The model under review builds one solid part; all positions refer to its coordinate system, in mm. Face numbers are marked on the shaded views. A direction names the side the tool comes from. Coordinates: 2 decimals unless noted, no trailing zeros. Order: outer loops, then holes, each group sorted by start corner. A loop starts at its lowest first (then second) coordinate and runs counter-clockwise, first axis right, second up. Notation, with made-up numbers: (-32, 30.5) -> (11, 30.5) arc R20 cw to (11, 48.5) -> close; hole circle Ø3 at (11.5, -10). An arc over 180 degrees is marked (long way). Answer as CSV lines item,"result". Start each with the question number.
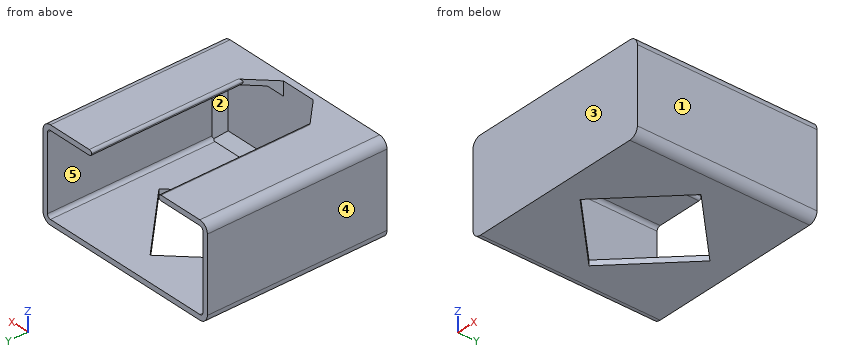
from build123d import *

# Parameters (mm, degrees)
RESSALTO_EXTRUS_O1_DEPTH = 1.5
RESSALTO_EXTRUS_O2_DEPTH = 40
ESBO_O4_W                = 18
ESBO_O4_H                = 3
CORTE_EXTRUS_O1_DEPTH    = 40
CORTE_EXTRUS_O2_DEPTH    = 8
CHANFRO1_SIZE            = 5
CHANFRO2_SIZE            = 2
FILETE2_START            = 6.5
FILETE2_DEPTH            = 35.5
FILETE2_START_2          = -3
FILETE2_2_DEPTH          = 1.232233047
FILETE3_START            = 6.5
FILETE3_DEPTH            = 35.5
FILETE3_START_2          = 1.767766953
FILETE3_2_DEPTH          = 1.232233047


with BuildPart() as part:
    # Esboço1 → Ressalto-extrusão1 (new body)
    with BuildSketch(Plane(origin=(0, 0, 0), x_dir=(1, 0, 0), z_dir=(0, 1, 0))):
        with BuildLine():
            Line((-20, -10.5), (20, -10.5))
            ThreePointArc((20, -10.5), (21.414213562, -9.914213562), (22, -8.5))
            Line((22, -8.5), (22, 8.5))
            ThreePointArc((22, 8.5), (21.414213562, 9.914213562), (20, 10.5))
            Line((20, 10.5), (-20, 10.5))
            ThreePointArc((-20, 10.5), (-21.414213562, 9.914213562), (-22, 8.5))
            Line((-22, 8.5), (-22, -8.5))
            ThreePointArc((-22, -8.5), (-21.414213562, -9.914213562), (-20, -10.5))
        make_face()
    extrude(amount=RESSALTO_EXTRUS_O1_DEPTH)

    # Esboço3 → Ressalto-extrusão2 (add)
    with BuildSketch(Plane(origin=(0, 1.5, 0), x_dir=(1, 0, 0), z_dir=(0, 1, 0))):
        with BuildLine():
            Line((-20, -10.5), (20, -10.5))
            ThreePointArc((20, -10.5), (21.414213562, -9.914213562), (22, -8.5))
            Line((22, -8.5), (22, 8.5))
            ThreePointArc((22, 8.5), (21.414213562, 9.914213562), (20, 10.5))
            Line((20, 10.5), (-20, 10.5))
            ThreePointArc((-20, 10.5), (-21.414213562, 9.914213562), (-22, 8.5))
            Line((-22, 8.5), (-22, -8.5))
            ThreePointArc((-22, -8.5), (-21.414213562, -9.914213562), (-20, -10.5))
        make_face()
        with BuildLine():
            Line((-20, 9.3), (20, 9.3))
            ThreePointArc((20, 9.3), (20.565685425, 9.065685425), (20.8, 8.5))
            Line((20.8, 8.5), (20.8, -8.5))
            ThreePointArc((20.8, -8.5), (20.565685425, -9.065685425), (20, -9.3))
            Line((20, -9.3), (-20, -9.3))
            ThreePointArc((-20, -9.3), (-20.565685425, -9.065685425), (-20.8, -8.5))
            Line((-20.8, -8.5), (-20.8, 8.5))
            ThreePointArc((-20.8, 8.5), (-20.565685425, 9.065685425), (-20, 9.3))
        make_face(mode=Mode.SUBTRACT)
    extrude(amount=RESSALTO_EXTRUS_O2_DEPTH)

    # Esboço4 → Corte-extrusão1 (cut)
    with BuildSketch(Plane(origin=(0, 41.5, 0), x_dir=(1, 0, 0), z_dir=(0, 1, 0))):
        with Locations((0, -9.3)):
            Rectangle(ESBO_O4_W, ESBO_O4_H)
    extrude(amount=-CORTE_EXTRUS_O1_DEPTH, mode=Mode.SUBTRACT)

    # Esboço5 → Corte-extrusão2 (cut)
    with BuildSketch(Plane(origin=(0, 0, -10.5), x_dir=(-1, 0, 0), z_dir=(0, 0, -1))):
        Polygon((0, 5.75), (15, 20.75), (0, 35.75), (-15, 20.75), align=None)
    extrude(amount=-CORTE_EXTRUS_O2_DEPTH, mode=Mode.SUBTRACT)

    # Chanfro1
    chanfro1_edges = [part.edges().sort_by_distance(p)[0] for p in [
        (9, 1.5, 9.9),
        (-9, 1.5, 9.9),
    ]]
    chamfer(chanfro1_edges, length=CHANFRO1_SIZE)

    # Chanfro2
    # the kernel refuses this chamfer: 2 mm, written as the material it adds along each edge
    with BuildSketch(Plane(origin=(-1.143365976, 1.5, 9.3), x_dir=(0, 1, 0), z_dir=(1, 0, 0))) as chanfro2_piece_1_section:
        Polygon((CHANFRO2_SIZE, 0), (0, -CHANFRO2_SIZE), (0, 0), align=None)
    chanfro2_piece_1 = extrude(amount=26.286731952, mode=Mode.PRIVATE)
    chanfro2_piece_1 = split(chanfro2_piece_1, bisect_by=Plane(origin=(20.8, 1.5, 9.3), z_dir=(-1, 0, 0)), keep=Keep.TOP, mode=Mode.PRIVATE)
    chanfro2_piece_1 = split(chanfro2_piece_1, bisect_by=Plane(origin=(1.428317012, -1.071682988, 9.3), z_dir=(0.7071067811865476, -0.7071067811865476, 0)), keep=Keep.TOP, mode=Mode.PRIVATE)
    add(chanfro2_piece_1)
    with BuildSketch(Plane(origin=(20.8, 1.5, -13.643365976), x_dir=(0, 1, 0), z_dir=(0, 0, 1))) as chanfro2_piece_2_section:
        Polygon((CHANFRO2_SIZE, 0), (0, CHANFRO2_SIZE), (0, 0), align=None)
    chanfro2_piece_2 = extrude(amount=27.286731952, mode=Mode.PRIVATE)
    chanfro2_piece_2 = split(chanfro2_piece_2, bisect_by=Plane(origin=(20.8, 1.5, -9.3), z_dir=(0, 0, 1)), keep=Keep.TOP, mode=Mode.PRIVATE)
    chanfro2_piece_2 = split(chanfro2_piece_2, bisect_by=Plane(origin=(20.8, 1.5, 9.3), z_dir=(0, 0, -1)), keep=Keep.TOP, mode=Mode.PRIVATE)
    add(chanfro2_piece_2)
    with BuildSketch(Plane(origin=(-25.143365976, 1.5, 9.3), x_dir=(0, 1, 0), z_dir=(1, 0, 0))) as chanfro2_piece_3_section:
        Polygon((CHANFRO2_SIZE, 0), (0, -CHANFRO2_SIZE), (0, 0), align=None)
    chanfro2_piece_3 = extrude(amount=26.286731952, mode=Mode.PRIVATE)
    chanfro2_piece_3 = split(chanfro2_piece_3, bisect_by=Plane(origin=(-20.8, 1.5, 9.3), z_dir=(1, 0, 0)), keep=Keep.TOP, mode=Mode.PRIVATE)
    chanfro2_piece_3 = split(chanfro2_piece_3, bisect_by=Plane(origin=(-14.571682988, 12.071682988, 9.3), z_dir=(-0.7071067811865476, -0.7071067811865476, 0)), keep=Keep.TOP, mode=Mode.PRIVATE)
    add(chanfro2_piece_3)
    with BuildSketch(Plane(origin=(-20.8, 1.5, 13.643365976), x_dir=(0, 1, 0), z_dir=(0, 0, -1))) as chanfro2_piece_4_section:
        Polygon((CHANFRO2_SIZE, 0), (0, CHANFRO2_SIZE), (0, 0), align=None)
    chanfro2_piece_4 = extrude(amount=27.286731952, mode=Mode.PRIVATE)
    chanfro2_piece_4 = split(chanfro2_piece_4, bisect_by=Plane(origin=(-20.8, 1.5, -9.3), z_dir=(0, 0, 1)), keep=Keep.TOP, mode=Mode.PRIVATE)
    chanfro2_piece_4 = split(chanfro2_piece_4, bisect_by=Plane(origin=(-20.8, 1.5, 9.3), z_dir=(0, 0, -1)), keep=Keep.TOP, mode=Mode.PRIVATE)
    add(chanfro2_piece_4)
    with BuildSketch(Plane(origin=(-25.143365976, 1.5, -9.3), x_dir=(0, 1, 0), z_dir=(1, 0, 0))) as chanfro2_piece_5_section:
        Polygon((CHANFRO2_SIZE, 0), (0, CHANFRO2_SIZE), (0, 0), align=None)
    chanfro2_piece_5 = extrude(amount=50.286731952, mode=Mode.PRIVATE)
    chanfro2_piece_5 = split(chanfro2_piece_5, bisect_by=Plane(origin=(20.8, 1.5, -9.3), z_dir=(-1, 0, 0)), keep=Keep.TOP, mode=Mode.PRIVATE)
    chanfro2_piece_5 = split(chanfro2_piece_5, bisect_by=Plane(origin=(-20.8, 1.5, -9.3), z_dir=(1, 0, 0)), keep=Keep.TOP, mode=Mode.PRIVATE)
    add(chanfro2_piece_5)
    with BuildSketch(Plane(origin=(-20, 1.5, -8.5), x_dir=(-1, 0, 0), z_dir=(0, 0, 1))) as chanfro2_piece_6_section:
        Polygon((0.8, -CHANFRO2_SIZE), (0, -1.2), (0, 0), (0.8, 0), align=None)
    chanfro2_piece_6 = revolve(axis=Axis((-20, 1.5, -8.5), (0, -1, 0)), revolution_arc=90, mode=Mode.PRIVATE)
    chanfro2_piece_6 = split(chanfro2_piece_6, bisect_by=Plane(origin=(-19.4, 2.1, -8.5), z_dir=(-0.7071067811865476, -0.7071067811865476, 0)), keep=Keep.TOP, mode=Mode.PRIVATE)
    add(chanfro2_piece_6)
    with BuildSketch(Plane(origin=(-20, 1.5, -8.5), x_dir=(-1, 0, 0), z_dir=(0, 0, 1))) as chanfro2_piece_7_section:
        Polygon((0.8, -CHANFRO2_SIZE), (0, -1.2), (0, 0), (0.8, 0), align=None)
    chanfro2_piece_7 = revolve(axis=Axis((-20, 1.5, -8.5), (0, -1, 0)), revolution_arc=90, mode=Mode.PRIVATE)
    chanfro2_piece_7 = split(chanfro2_piece_7, bisect_by=Plane(origin=(-20, 2.1, -7.9), z_dir=(0, -0.7071067811865476, -0.7071067811865476)), keep=Keep.TOP, mode=Mode.PRIVATE)
    add(chanfro2_piece_7)
    with BuildSketch(Plane(origin=(20, 1.5, -8.5), x_dir=(0, 0, -1), z_dir=(-1, 0, 0))) as chanfro2_piece_8_section:
        Polygon((0.8, -CHANFRO2_SIZE), (0, -1.2), (0, 0), (0.8, 0), align=None)
    chanfro2_piece_8 = revolve(axis=Axis((20, 1.5, -8.5), (0, -1, 0)), revolution_arc=90, mode=Mode.PRIVATE)
    chanfro2_piece_8 = split(chanfro2_piece_8, bisect_by=Plane(origin=(20, 2.1, -7.9), z_dir=(0, -0.7071067811865476, -0.7071067811865476)), keep=Keep.TOP, mode=Mode.PRIVATE)
    add(chanfro2_piece_8)
    with BuildSketch(Plane(origin=(20, 1.5, -8.5), x_dir=(0, 0, -1), z_dir=(-1, 0, 0))) as chanfro2_piece_9_section:
        Polygon((0.8, -CHANFRO2_SIZE), (0, -1.2), (0, 0), (0.8, 0), align=None)
    chanfro2_piece_9 = revolve(axis=Axis((20, 1.5, -8.5), (0, -1, 0)), revolution_arc=90, mode=Mode.PRIVATE)
    chanfro2_piece_9 = split(chanfro2_piece_9, bisect_by=Plane(origin=(19.4, 2.1, -8.5), z_dir=(0.7071067811865476, -0.7071067811865476, 0)), keep=Keep.TOP, mode=Mode.PRIVATE)
    add(chanfro2_piece_9)
    with BuildSketch(Plane(origin=(-20, 1.5, 8.5), x_dir=(0, 0, 1), z_dir=(1, 0, 0))) as chanfro2_piece_10_section:
        Polygon((0.8, -CHANFRO2_SIZE), (0, -1.2), (0, 0), (0.8, 0), align=None)
    chanfro2_piece_10 = revolve(axis=Axis((-20, 1.5, 8.5), (0, -1, 0)), revolution_arc=90, mode=Mode.PRIVATE)
    chanfro2_piece_10 = split(chanfro2_piece_10, bisect_by=Plane(origin=(-20, 2.1, 7.9), z_dir=(0, -0.7071067811865476, 0.7071067811865476)), keep=Keep.TOP, mode=Mode.PRIVATE)
    add(chanfro2_piece_10)
    with BuildSketch(Plane(origin=(-20, 1.5, 8.5), x_dir=(0, 0, 1), z_dir=(1, 0, 0))) as chanfro2_piece_11_section:
        Polygon((0.8, -CHANFRO2_SIZE), (0, -1.2), (0, 0), (0.8, 0), align=None)
    chanfro2_piece_11 = revolve(axis=Axis((-20, 1.5, 8.5), (0, -1, 0)), revolution_arc=90, mode=Mode.PRIVATE)
    chanfro2_piece_11 = split(chanfro2_piece_11, bisect_by=Plane(origin=(-19.4, 2.1, 8.5), z_dir=(-0.7071067811865476, -0.7071067811865476, 0)), keep=Keep.TOP, mode=Mode.PRIVATE)
    add(chanfro2_piece_11)
    with BuildSketch(Plane(origin=(20, 1.5, 8.5), x_dir=(1, 0, 0), z_dir=(0, 0, -1))) as chanfro2_piece_12_section:
        Polygon((0.8, -CHANFRO2_SIZE), (0, -1.2), (0, 0), (0.8, 0), align=None)
    chanfro2_piece_12 = revolve(axis=Axis((20, 1.5, 8.5), (0, -1, 0)), revolution_arc=90, mode=Mode.PRIVATE)
    chanfro2_piece_12 = split(chanfro2_piece_12, bisect_by=Plane(origin=(19.4, 2.1, 8.5), z_dir=(0.7071067811865476, -0.7071067811865476, 0)), keep=Keep.TOP, mode=Mode.PRIVATE)
    add(chanfro2_piece_12)
    with BuildSketch(Plane(origin=(20, 1.5, 8.5), x_dir=(1, 0, 0), z_dir=(0, 0, -1))) as chanfro2_piece_13_section:
        Polygon((0.8, -CHANFRO2_SIZE), (0, -1.2), (0, 0), (0.8, 0), align=None)
    chanfro2_piece_13 = revolve(axis=Axis((20, 1.5, 8.5), (0, -1, 0)), revolution_arc=90, mode=Mode.PRIVATE)
    chanfro2_piece_13 = split(chanfro2_piece_13, bisect_by=Plane(origin=(20, 2.1, 7.9), z_dir=(0, -0.7071067811865476, 0.7071067811865476)), keep=Keep.TOP, mode=Mode.PRIVATE)
    add(chanfro2_piece_13)

    # Filete2: read off the stored shape, not the designer's step
    # Filete2 outline → Filete2 (cut)
    with BuildSketch(Plane(origin=(0, 0, 0), x_dir=(1, 0, 0), z_dir=(0, 1, 0)).offset(FILETE2_START)):
        with BuildLine():
            ThreePointArc((-9.6, -9.3), (-9.175735931, -9.475735931), (-9, -9.9))
            Line((-9, -9.9), (-9, -9.3))
            Line((-9, -9.3), (-9.6, -9.3))
        make_face()
        with BuildLine():
            ThreePointArc((-9, -9.9), (-9.175735931, -10.324264069), (-9.6, -10.5))
            Line((-9.6, -10.5), (-9, -10.5))
            Line((-9, -10.5), (-9, -9.9))
        make_face()
    extrude(amount=FILETE2_DEPTH, mode=Mode.SUBTRACT)

    # Filete2 2 outline → Filete2 2 (add)
    with BuildSketch(Plane(origin=(0, 0, 0), x_dir=(0.7071067811865509, -0.707106781186544, 0), z_dir=(0.707106781186544, 0.707106781186551, 0)).offset(FILETE2_START_2)):
        with BuildLine():
            Line((-3.889087297, -7.3), (-6.717514421, -9.3))
            Line((-6.717514421, -9.3), (-11.808683246, -9.3))
            add(Edge.make_bspline(
                [(-11.808683246, -10.5), (-10.960155108, -10.5), (-10.960155108, -9.9), (-10.960155108, -9.3), (-11.808683246, -9.3)],
                knots=[1.570796327, 1.570796327, 1.570796327, 3.141592654, 3.141592654, 4.71238898, 4.71238898, 4.71238898], degree=2, weights=[1, 0.707106781, 1, 0.707106781, 1]))
            Line((-11.808683246, -10.5), (-3.889087297, -10.5))
            Line((-3.889087297, -10.5), (-3.889087297, -7.3))
        make_face()
    extrude(amount=FILETE2_2_DEPTH)

    # Filete3: read off the stored shape, not the designer's step
    # Filete3 outline → Filete3 (cut)
    with BuildSketch(Plane(origin=(0, 0, 0), x_dir=(1, 0, 0), z_dir=(0, 1, 0)).offset(FILETE3_START)):
        with BuildLine():
            Line((9, -10.5), (9.6, -10.5))
            ThreePointArc((9.6, -10.5), (9.175735931, -10.324264069), (9, -9.9))
            Line((9, -9.9), (9, -10.5))
        make_face()
        with BuildLine():
            Line((9, -9.3), (9, -9.9))
            ThreePointArc((9, -9.9), (9.175735931, -9.475735931), (9.6, -9.3))
            Line((9.6, -9.3), (9, -9.3))
        make_face()
    extrude(amount=FILETE3_DEPTH, mode=Mode.SUBTRACT)

    # Filete3 2 outline → Filete3 2 (add)
    with BuildSketch(Plane(origin=(0, 0, 0), x_dir=(0.7071067811865509, 0.707106781186544, 0), z_dir=(0.707106781186544, -0.707106781186551, 0)).offset(FILETE3_START_2)):
        with BuildLine():
            Line((11.808683246, 10.5), (3.889087297, 10.5))
            Line((3.889087297, 10.5), (3.889087297, 7.3))
            Line((3.889087297, 7.3), (6.717514421, 9.3))
            Line((6.717514421, 9.3), (11.808683246, 9.3))
            add(Edge.make_bspline(
                [(11.808683246, 9.3), (10.960155108, 9.3), (10.960155108, 9.9), (10.960155108, 10.5), (11.808683246, 10.5)],
                knots=[4.71238898, 4.71238898, 4.71238898, 6.283185307, 6.283185307, 7.853981634, 7.853981634, 7.853981634], degree=2, weights=[1, 0.707106781, 1, 0.707106781, 1]))
        make_face()
    extrude(amount=FILETE3_2_DEPTH)


solid = part.part
1) Consider section A-A (x = 2.5). Give the boundary of the cut face in (y, z), plus the area to 3 significant figures.
2) Wall thickness on L1, parallel to X at y = 5.5, z = -8.5; L2, parallel to Z at x = 12, y = 14; L3, parallel to Y at x = 6.5, z = 3.5: over which ranges is each line inside the solid? List them lowest first. Write a range as [from, to].
3) Mouldability with a two-part tool opening along X and no side actions: class the marked faces 3, 4 and 5 as released by +X, released by -X, zero draft, split by the parting line, or undercut.
4) Consider section C-C (y = 39). Give the boundary of the cut face in (x, z).
5) Tool access review of the marked faces 1 and 2: name each direction out of +Z, -Z, +X, -X, +Y, -Y from which nothing blocks a thin tool from reaching the whole face with its end or side.
6) Consider section B-B (y = 18). Give the boundary of the cut face in (x, z).
7) Insertion check: pin 1 Ø9 at (x, z) = (7, 3) entering from +Y; pin 2 Ø1 at (x, z) = (-8, 4) entering from -Y; pin 3 Ø10 at (x, y) = (-1, 9) entering from +Z; pin 4 Ø6 at (x, z) = (14.5, -2) entering from +Y. Each pin has a flat end and moves straight along its axis. Give the tip position at first contact, or say it passes through.
8) Consider section D-D (x = 8). Give the boundary of the cut face in (y, z).
Result:
1,outline,"(0, -10.5) -> (8.25, -10.5) -> (8.25, -9.3) -> (3.5, -9.3) -> (1.5, -7.3) -> (1.5, 10.5) -> (0, 10.5) -> close; (33.25, -10.5) -> (41.5, -10.5) -> (41.5, -9.3) -> (33.25, -9.3) -> close"
1,area,"51.5 mm2"
2,L1,"[-22, -20.8], [20.8, 22]"
2,L2,"[-10.5, -9.3], [9.3, 10.5]"
2,L3,"[0, 1.5]"
3,face 3,"zero draft"
3,face 4,"released by -X"
3,face 5,"undercut"
4,outline,"(-22, -8.5) arc R2 ccw to (-20, -10.5) -> (20, -10.5) arc R2 ccw to (22, -8.5) -> (22, 8.5) arc R2 ccw to (20, 10.5) -> (9.6, 10.5) arc R0.6 ccw to (9.6, 9.3) -> (20, 9.3) arc R0.8 cw to (20.8, 8.5) -> (20.8, -8.5) arc R0.8 cw to (20, -9.3) -> (-20, -9.3) arc R0.8 cw to (-20.8, -8.5) -> (-20.8, 8.5) arc R0.8 cw to (-20, 9.3) -> (-9.6, 9.3) arc R0.6 ccw to (-9.6, 10.5) -> (-20, 10.5) arc R2 ccw to (-22, 8.5) -> close"
5,face 1,"+Z, -Z, +X, +Y, -Y"
5,face 2,"+Y"
6,outline,"(-22, -8.5) arc R2 ccw to (-20, -10.5) -> (-12.25, -10.5) -> (-12.25, -9.3) -> (-20, -9.3) arc R0.8 cw to (-20.8, -8.5) -> (-20.8, 8.5) arc R0.8 cw to (-20, 9.3) -> (-9.6, 9.3) arc R0.6 ccw to (-9.6, 10.5) -> (-20, 10.5) arc R2 ccw to (-22, 8.5) -> close; (9.6, 9.3) -> (20, 9.3) arc R0.8 cw to (20.8, 8.5) -> (20.8, -8.5) arc R0.8 cw to (20, -9.3) -> (12.25, -9.3) -> (12.25, -10.5) -> (20, -10.5) arc R2 ccw to (22, -8.5) -> (22, 8.5) arc R2 ccw to (20, 10.5) -> (9.6, 10.5) arc R0.6 ccw to start"
7,pin 1,"y = 1.7"
7,pin 2,"y = 0"
7,pin 3,"z = -9.3"
7,pin 4,"y = 1.5"
8,outline,"(0, -10.5) -> (13.75, -10.5) -> (13.75, -9.3) -> (3.5, -9.3) -> (1.5, -7.3) -> (1.5, 7.3) -> (3.5, 9.3) -> (5.5, 9.3) -> (5.5, 10.5) -> (0, 10.5) -> close; (27.75, -10.5) -> (41.5, -10.5) -> (41.5, -9.3) -> (27.75, -9.3) -> close"
